```python
from build123d import *

# Parameters (mm, degrees)
F0_W     = 30
F0_H     = 30
F1_DEPTH = 15
F2_R     = 5
F3_DEPTH = 30


# Not quite as in the source:
# - a feature of the source that left no trace in its solid (it failed there, or was rolled back) is left out


with BuildPart() as f1:
    # F0 (on Top) → F1 (new body, symmetric)
    with BuildSketch(Plane.XY):
        Rectangle(F0_W, F0_H)
    extrude(amount=F1_DEPTH, both=True)

    # F2 (on face) → F3 (join)
    with BuildSketch(Plane.XZ.offset(15)):
        Circle(F2_R)
    extrude(amount=F3_DEPTH)


solid = f1.part
```
Input: part model. Units: mm. Frame: model coordinates. A direction names the side the tool comes from. Round coordinates to 2 decimals unless told otherwise and drop trailing zeros. Loops run counter-clockwise (first coordinate to the right, second up) from the corner with the lowest first, then second, coordinate; pieces in that order, holes last. Notation, with made-up numbers: (17, 65) -> (55, 65) arc R31 ccw to (55, 97) -> close; hole circle Ø8 at (-13, 43). An arc over 180 degrees is marked (long way). Use one line per item in the form item = value. Start each with the question number.
Item 1: Section query B-B on z = 0. Return the cut outline in (x, y), then the cut area to 3 significant figures.
Item 2: Section query D-D on z = 7.25. Return the cut outline in (x, y), then the cut area to 3 significant figures.
Item 3: Section query C-C on y = -30. Return the cut outline in (x, z).
Item 4: Material intervals for L1, parallel to Y at x = -10.5, z = 1.75; L2, parallel to Z at x = -0.5, y = -37.5, sorted ascending. Write a range as from..to.
Item 5: Set-up query: faces 1 (the face through (-1.08, -29.79, -4.88)), 2 (the face through (0, 0, 15)). Return all of +Z, -Z, +X, -X, +Y, -Y with unobstructed straight access to the full face (end or side cutting, diameter ignored); none if empty.
Item 6: Section query A-A on x = -3. Return the cut outline in (y, z), then the cut area to 3 significant figures.
Item 7: Contact query for flat-ended pins moving along their axis: pin 1 Ø4 at (y, z) = (-31.5, -2) entering from +X; pin 2 Ø3 at (y, z) = (-22, 1.5) entering from -X; pin 3 Ø2 at (x, y) = (5, -17) entering from -Z. Output: stop coordinate, or through.
Ans:
q1.outline = (-15, -15) -> (-5, -15) -> (-5, -45) -> (5, -45) -> (5, -15) -> (15, -15) -> (15, 15) -> (-15, 15) -> close
q1.area = 1,200 mm^2
q2.outline = (-15, -15) -> (15, -15) -> (15, 15) -> (-15, 15) -> close
q2.area = 900 mm^2
q3.outline = circle Ø10 at (0, 0)
q4.L1 = -15..15
q4.L2 = -4.97..4.97
q5.face_1 = -Y
q5.face_2 = +Z, +X, -X, +Y, -Y
q6.outline = (-45, -4) -> (-15, -4) -> (-15, -15) -> (15, -15) -> (15, 15) -> (-15, 15) -> (-15, 4) -> (-45, 4) -> close
q6.area = 1,140 mm^2
q7.pin_1 = 5
q7.pin_2 = -5
q7.pin_3 = -3
